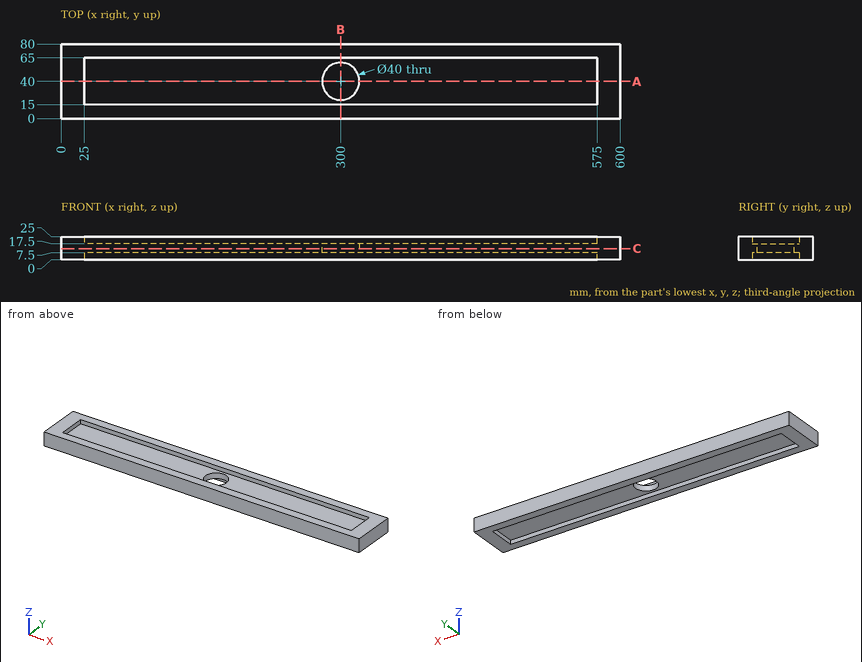
Geometry check sheet. Reference: drawing and pictorial views, mm from the part's lowest x, y, z. Give positions to 0.01 mm unless a question says otherwise; leave off trailing zeros. Order: outer loops, then holes, each group sorted by start corner. A loop starts at its lowest first (then second) coordinate and runs counter-clockwise, first axis right, second up. Notation, with made-up numbers: M -23,79 L 31,79 A14 cw 31,88 Z; hole C -28,-34.5 d6. An arc over 180 degrees is marked long. Answer in a Markdown table with one row per item. Add a question column.
Q1. Thickness scan on L1, parallel to X at y = 62, z = 22.75; L2, parallel to Y at x = 300, z = 12.5; L3, parallel to Y at x = 71.5, z = 20. Record the ranges inside material, lowest first.
Q2. Sectioned sample at B-B, the plane x = 300. Record the boundary of the cut face in (y, z).
Q3. Gauge pin test, flat ends, axial feed: pin 1 Ø25 at (x, y) = (248, 38.5) entering from -Z; pin 2 Ø2 at (x, y) = (475, 59) entering from +Z. Record the tip position at first contact, or that the pin passes through.
Q4. Sectioned sample at C-C, the plane z = 12. Record the boundary of the cut face in (x, y), and give its area (3 significant figures).
Q5. Sectioned sample at A-A, the plane y = 40. Record the boundary of the cut face in (x, z), and give its area (3 significant figures).
Verdict:
| question | item | result |
|---|---|---|
| 1 | L1 | 0 to 25, 575 to 600 |
| 1 | L2 | 0 to 20, 60 to 80 |
| 1 | L3 | 0 to 15, 65 to 80 |
| 2 | outline | M 0,0 L 15,0 L 15,7.5 L 20,7.5 L 20,17.5 L 15,17.5 L 15,25 L 0,25 Z; M 60,7.5 L 65,7.5 L 65,0 L 80,0 L 80,25 L 65,25 L 65,17.5 L 60,17.5 Z |
| 3 | pin 1 | z = 7.5 |
| 3 | pin 2 | z = 17.5 |
| 4 | outline | M 0,0 L 600,0 L 600,80 L 0,80 Z; hole C 300,40 d40 |
| 4 | area | 46,700 mm² |
| 5 | outline | M 0,0 L 25,0 L 25,7.5 L 280,7.5 L 280,17.5 L 25,17.5 L 25,25 L 0,25 Z; M 320,7.5 L 575,7.5 L 575,0 L 600,0 L 600,25 L 575,25 L 575,17.5 L 320,17.5 Z |
| 5 | area | 6,350 mm² |
